Autodesk Fusion 360 part; units mm, degrees
sketch "Sketch1" plane through (0, 0, 0) normal (0, 1, 0) x (1, 0, 0)
  line L0 (0, 0) -> (5, 0)
  line L1 (5, 0) -> (5, -10)
  line L2 (5, -10) -> (0, -10)
  line L3 (0, -10) -> (0, 0)
  line L4 (0, -1) -> (5, -1)
  line L5 (0, -3) -> (5, -3)
  line L6 (0, -4) -> (5, -4)
  circle A0 centre (2.5, -7) radius 1
  dimension "d1" = 10
  dimension "d2" = 5
  dimension "d3" = 2
  dimension "d4" = 1
  dimension "d5" = 1
  dimension "d6" = 2
ref_plane "WorkPlane1" through (2.5, 5, 3.5) normal (0, 1, 0) x (1, 0, 0)
ref_plane "WorkPlane2" through (2.5, 5, 0.5) normal (0, 1, 0) x (1, 0, 0)
ref_plane "WorkPlane3" through (2.5, 1, 2) normal (0, 1, 0) x (1, 0, 0)
ref_plane "WorkPlane4" through (2.5, 1, 7) normal (0, 1, 0) x (1, 0, 0)
sketch "Sketch2" plane through (0, 0, 0) normal (1, 0, 0) x (0, 0, -1)
  line L0 (-1, 11) -> (-1, 1)
  line L1 (-1, 1) -> (-3, 1)
  line L2 (-3, 1) -> (-3, 11)
  line L3 (-3, 11) -> (-4, 11)
  line L4 (-4, 11) -> (-4, 1)
  line L5 (-4, 1) -> (-10, 1)
  line L6 (-10, 1) -> (-10, 0)
  line L7 (-10, 0) -> (0, 0)
  line L8 (0, 11) -> (-1, 11)
  line L9 (0, 0) -> (-10, 0)
  line L10 (0, 11) -> (0, 1)
  line L11 (0, 1) -> (0, 0)
  line L12 (0, 1) -> (0, 11)
  point P0 (-10, 0)
  dimension "d11" = 10
  dimension "d12" = 2
  dimension "d13" = 10
  dimension "d14" = 1
  dimension "d15" = 1
  dimension "d17" = 6
  dimension "d18" = 1
  dimension "d20" = 1
  dimension "d21" = 10
extrude "Extrude1" add sketch "Sketch2" along normal blind 5
extrude "Extrude2" cut sketch "Sketch1" along normal blind 1 contours A0
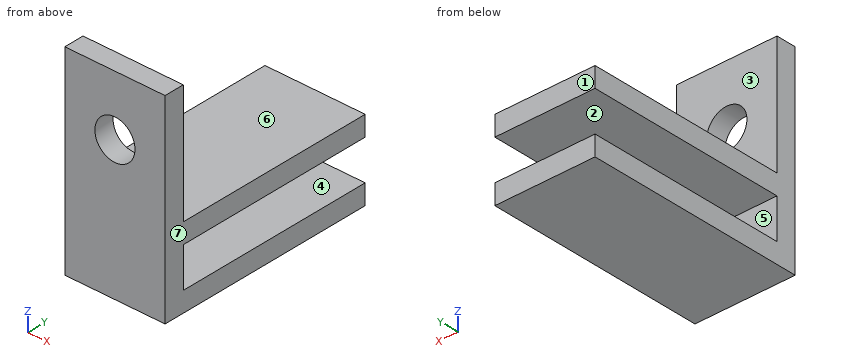
The listing builds one solid part. Answer for the finished solid, in the listing's coordinates (mm). Face numbers are marked on the shaded views. A direction names the side the tool comes from. Give positions to 0.01 mm unless a question says otherwise; leave off trailing zeros. Order: outer loops, then holes, each group sorted by start corner. A loop starts at its lowest first (then second) coordinate and runs counter-clockwise, first axis right, second up. Notation, with made-up numbers: (-21, 56) -> (34, 56) arc R30 cw to (34, 79) -> close; hole circle Ø10 at (30.5, 60.25). An arc over 180 degrees is marked (long way). Put each result on its own line as item: value.
Item 1: A cutting plane is placed at A-A on z = 7. Give the vertices of the cut face in (x, y).
Established:
outline: (0, 0) -> (1.5, 0) -> (1.5, 1) -> (0, 1) -> close; (3.5, 0) -> (5, 0) -> (5, 1) -> (3.5, 1) -> close
Item 2: A cutting plane is placed at B-B on x = 1.8. Give the vertices of the cut face in (y, z), plus the area to 3 significant figures.
Established:
outline: (0, 0) -> (11, 0) -> (11, 1) -> (1, 1) -> (1, 3) -> (11, 3) -> (11, 4) -> (1, 4) -> (1, 6.29) -> (0, 6.29) -> close; (0, 7.71) -> (1, 7.71) -> (1, 10) -> (0, 10) -> close
area: 28.6 mm^2
Item 3: A cutting plane is placed at D-D on x = 1. Give the vertices of the cut face in (y, z).
Established:
outline: (0, 0) -> (11, 0) -> (11, 1) -> (1, 1) -> (1, 3) -> (11, 3) -> (11, 4) -> (1, 4) -> (1, 10) -> (0, 10) -> close
Item 4: Given P1, Ø1.8, axis at x = 2.5, z = 7, coming from the +Y side, flat-ended and moving along its own axis, determine where the tip first touches the part or whether it passes through.
Established:
P1: passes through
Item 5: Straight lines are drawn through the part: line 1 (X direction, y = 0.75, z = 7); line 2 (Z direction, x = 2.5, y = 0.6); line 3 (Z direction, x = 3.5, y = 5). For each, find the intervals that lie inside material, in ascending order.
Established:
line 1: x = 0 to 1.5, 3.5 to 5
line 2: z = 0 to 6, 8 to 10
line 3: z = 0 to 1, 3 to 4
Item 6: For a pull along Z with two mould halves and no side action, classify the marked faces 4, 5, 6 and 7 as released by +Z, released by -Z, zero draft, split by the parting line, or undercut.
Established:
face 4: undercut
face 5: undercut
face 6: released by +Z
face 7: zero draft
Item 7: A cutting plane is placed at C-C on y = 3.5. Give the vertices of the cut face in (x, z).
Established:
outline: (0, 0) -> (5, 0) -> (5, 1) -> (0, 1) -> close; (0, 3) -> (5, 3) -> (5, 4) -> (0, 4) -> close
Item 8: For the marked faces 1, 2 and 3, determine the directions among +Z, -Z, +X, -X, +Y, -Y from which every point of the face is accessible in a straight line to the end or side of a thin tool.
Established:
face 1: +Z, -Z, +X, -X, +Y
face 2: +X, -X, +Y
face 3: +Z, +X, -X, +Y
